Part print with two shaded views. Sizes in mm from the minimum x, y, z corner. A direction names the side the tool comes from. Round coordinates to 2 decimals unless told otherwise and drop trailing zeros. Loops run counter-clockwise (first coordinate to the right, second up) from the corner with the lowest first, then second, coordinate; pieces in that order, holes last.
(1) Flat gauge pins, fed straight in: pin 1 (24 mm diameter, centred on x = 59.5, z = 118.5, fed in from -Y); pin 2 (15 mm diameter, centred on x = 33, z = 142.5, fed in from +Y); pin 3 (1.6 mm diameter, centred on x = 69, y = 52.5, fed in from +Z). Where does each tip first touch, or does it go through?
(2) Cut at A-A on x = 35.25. List the corners of the cut face in (y, z), then the cut area to 3 significant figures.
(3) Cut at C-C on z = 118.5. List the corners of the cut face in (x, y).
(4) Cut at B-B on y = 40.5. List the corners of the cut face in (x, z).
(5) Mould opens along Z. For the marked faces 1, 2 and 3 say: +Z half, -Z half, draft (parallel to the pull), parting line (faces both ways), or undercut.
(6) Cut at D-D on x = 63. List the corners of the cut face in (y, z).
(7) Tool access for the marked faces 4, 5, 6 and 7: list every direction of +Z, -Z, +X, -X, +Y, -Y with a clear straight run to the whole face (end or side of a thin tool).
(8) Probe probe 1 along Z at (x, y) = (35, 30); probe 2 along X at (y, z) = (9.75, 20); probe 3 along X at (y, z) = (67.9, 140). List the from-to ranges inside material, lowest first.
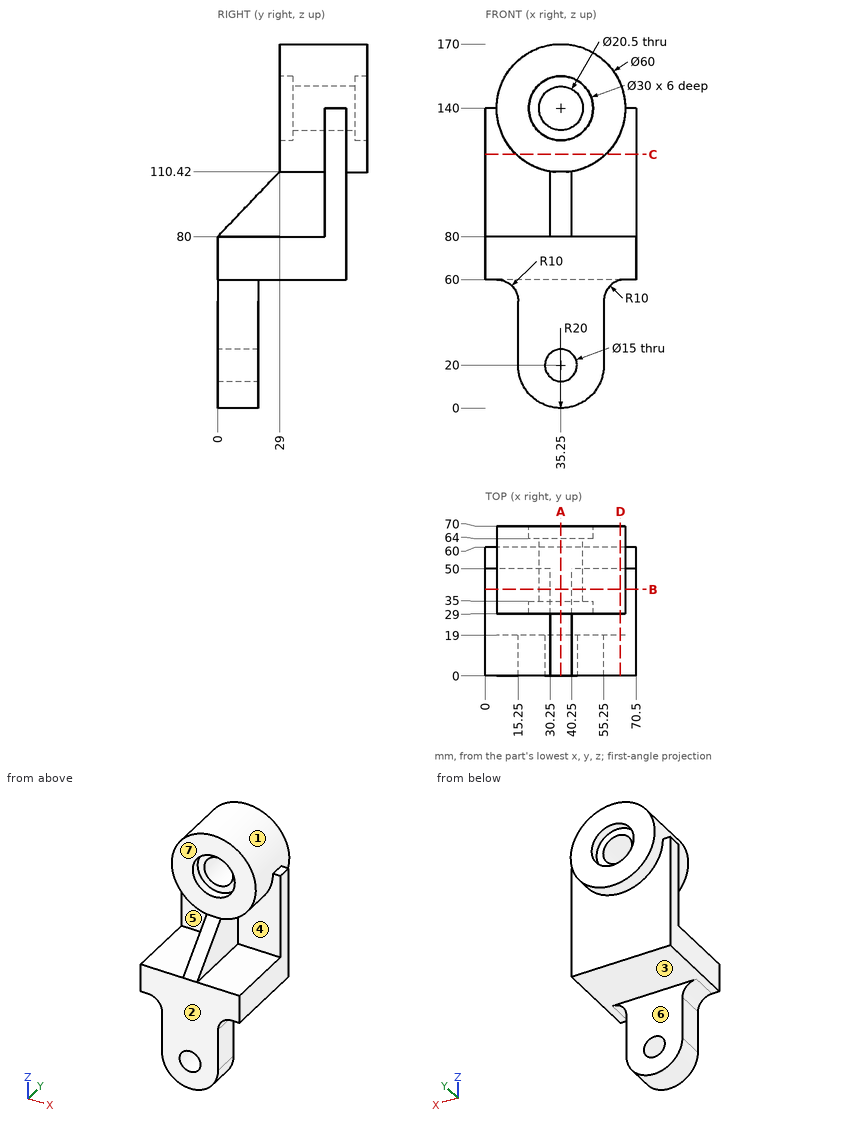
Final values:
1. pin 1: stops at y = 29
1. pin 2: stops at y = 64
1. pin 3: stops at z = 140
2. outline: (0, 0) - (19, 0) - (19, 12.5) - (0, 12.5) - close; (0, 27.5) - (19, 27.5) - (19, 60) - (60, 60) - (60, 110) - (70, 110) - (70, 125) - (64, 125) - (64, 129.75) - (35, 129.75) - (35, 125) - (29, 125) - (29, 110.42) - (0, 80) - close; (29, 155) - (35, 155) - (35, 150.25) - (64, 150.25) - (64, 155) - (70, 155) - (70, 170) - (29, 170) - close
2. area: 4,930 mm2
3. outline: (0, 50) - (14.33, 50) - (14.33, 29) - (56.17, 29) - (56.17, 50) - (70.5, 50) - (70.5, 60) - (56.17, 60) - (56.17, 70) - (14.33, 70) - (14.33, 60) - (0, 60) - close
4. outline: (0, 60) - (70.5, 60) - (70.5, 80) - (40.25, 80) - (40.25, 110.42) arc R30 ccw (long way) to (30.25, 110.42) - (30.25, 80) - (0, 80) - close; hole circle Ø20.5 at (35.25, 140)
5. face 1: undercut
5. face 2: draft
5. face 3: -Z half
6. outline: (0, 59.74) - (19, 59.74) - (19, 60) - (60, 60) - (60, 128.6) - (70, 128.6) - (70, 151.4) - (29, 151.4) - (29, 128.6) - (50, 128.6) - (50, 80) - (0, 80) - close
7. face 4: +X, -Y
7. face 5: -X, -Y
7. face 6: -Z, +X, -X, +Y
7. face 7: +Z, +X, -X, -Y
8. probe 1: z = 60 to 125, 155 to 170
8. probe 2: x = 15.25 to 27.75, 42.75 to 55.25
8. probe 3: x = 5.25 to 20.25, 50.25 to 65.25
